The listing builds one solid part. Answer for the finished solid, in the listing's coordinates (mm). Face numbers are marked on the shaded views. Give positions to 0.01 mm unless a question says otherwise; leave off trailing zeros. Put each result on its own line as item: value. Start each with the question number.
1) For a pull along X with two mould halves and no side action, classify the marked faces 1, 2 and 3 as released by +X, released by -X, zero draft, split by the parting line, or undercut.
2) Find the intervals of material crossed by line 1 along Y through (x, z) = (93, -6.5); line 2 along Y through (x, z) = (51, 3); line 3 along Z through (x, y) = (71, -6), in increasing order. Write a range as from..to.
3) Flat-ended cylindrical pins translate along their axes: pin 1 Ø2 at (x, z) = (100.5, -0.5) entering from -Y; pin 2 Ø4 at (x, z) = (111, -8) entering from -Y; pin 3 Ø8 at (x, y) = (91.5, 1) entering from +Z. Find the tip coordinate at first contact, or state that the pin passes through.
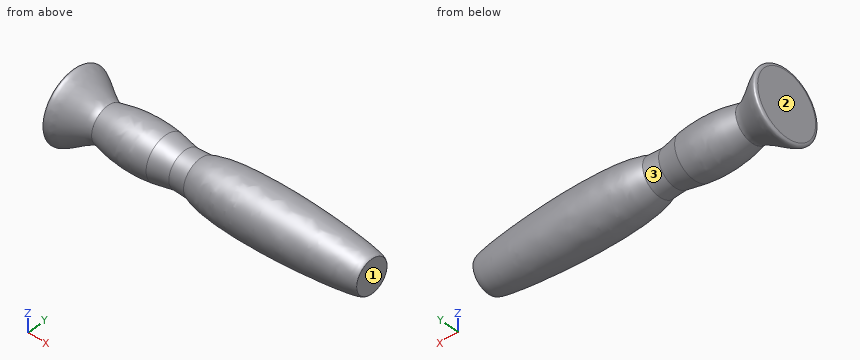
from build123d import *


with BuildPart() as f1:
    # F0 (on Front) → F1 (revolve)
    with BuildSketch(Plane.XZ):
        with BuildLine():
            Line((0, 0), (136, 0))
            Line((136, 0), (136, 7.5668375939))
            add(Edge.make_bspline(
                [(57.932120328, 8.4838647993), (74.0178674459, 15.4621964321), (136, 9.8442165181), (136, 7.5668375939)],
                knots=[0, 0, 0, 0, 78.073265433, 78.073265433, 78.073265433, 78.073265433], degree=3))
            Line((57.932120328, 8.4838647993), (50.9394065873, 8.1645615891))
            Line((50.9394065873, 8.1645615891), (42.0975312591, 9.8442165181))
            add(Edge.make_bspline(
                [(15.7956126534, 8.215207171), (26.520403102, 11.1532055438), (36.1618974445, 10.6971871138), (42.0975312591, 9.8442165181)],
                knots=[0, 0, 0, 0, 26.3523166684, 26.3523166684, 26.3523166684, 26.3523166684], degree=3))
            add(Edge.make_bspline(
                [(0, 14.5), (0, 19.5479989052), (11.198640801, 8.215207171), (15.7956126534, 8.215207171)],
                knots=[0, 0, 0, 0, 17, 17, 17, 17], degree=3))
            Line((0, 14.5), (0, 0))
        make_face()
    revolve(axis=Axis((68, 0, 0), (-1, 0, 0)))


solid = f1.part
Reply:
1. face 1: released by +X
1. face 2: released by -X
1. face 3: undercut
2. line 1: y = -9.87..9.87
2. line 2: y = -7.6..7.6
2. line 3: z = -9.43..9.43
3. pin 1: stops at y = -11.64
3. pin 2: stops at y = -9.27
3. pin 3: stops at z = 11.87
